Could you check a few things on this model? Use its own coordinates, in mm. A direction names the side the tool comes from. Round coordinates to 2 decimals unless told otherwise and drop trailing zeros. Loops run counter-clockwise (first coordinate to the right, second up) from the corner with the lowest first, then second, coordinate; pieces in that order, holes last.
from build123d import *

# Parameters (mm, degrees)
SKETCH_1_W                = 47
SKETCH_1_H                = 50
EXTRUDE_1_DEPTH           = 100
SKETCH_2_W                = 43
SKETCH_2_H                = 46
CUT_EXTRUDE_1_DEPTH       = 122.280666225
HOLE_WIZARD_1_D           = 2.4
HOLE_WIZARD_1_CSINK_D     = 4.5
HOLE_WIZARD_1_CSINK_ANGLE = 90
SKETCH_31_W               = 4
SKETCH_31_H               = 25
EXTRUDE_4_DEPTH           = 37
SKETCH_32_R               = 5
CUT_EXTRUDE_2_DEPTH       = 4
SKETCH_33_R               = 1.9
EXTRUDE_5_DEPTH           = 1.6
SKETCH_34_R               = 1.05
CUT_EXTRUDE_3_DEPTH       = 101.189819842
SKETCH_35_W               = 68
SKETCH_35_H               = 4
EXTRUDE_6_DEPTH           = 35
CUT_EXTRUDE_4_REACH       = 123.281
SKETCH_36_R               = 1.25
CUT_EXTRUDE_5_REACH       = 123.281
CUT_EXTRUDE_6_REACH       = 123.281
SKETCH_39_R               = 2.5
CUT_EXTRUDE_7_DEPTH       = 1.5
CUT_EXTRUDE_8_DEPTH       = 2
CUT_EXTRUDE_9_REACH       = 122.47
SKETCH_41_R               = 1.5
SKETCH_42_R               = 1.5
CUT_EXTRUDE_10_DEPTH      = 2
RIB_2_REACH               = 99.933
SKETCH_46_WALL_W          = 251.717080448
SKETCH_46_WALL_H          = 2
RIB_3_REACH               = 100.118
SKETCH_47_WALL_W          = 252.08841221
SKETCH_47_WALL_H          = 2
SKETCH_48_W               = 2
SKETCH_48_H               = 15
EXTRUDE_7_DEPTH           = 20
CUT_EXTRUDE_11_REACH      = 105.589


with BuildPart() as part:
    # 草图1 → 凸台-拉伸1 (new body)
    with BuildSketch(Plane(origin=(0, 0, 0), x_dir=(0, 0, -1), z_dir=(1, 0, 0))):
        with Locations((-23.5, 25)):
            Rectangle(SKETCH_1_W, SKETCH_1_H)
    extrude(amount=-EXTRUDE_1_DEPTH)

    # 草图2 → 切除-拉伸1 (cut, through all)
    with BuildSketch(Plane(origin=(0, 0, 0), x_dir=(0, 0, -1), z_dir=(1, 0, 0))):
        with Locations((-25.5, 23)):
            Rectangle(SKETCH_2_W, SKETCH_2_H)
    extrude(amount=-CUT_EXTRUDE_1_DEPTH, mode=Mode.SUBTRACT)

    # 打孔尺寸(%根据十字)槽沉头木螺钉的类型1 (through all)
    with Locations(Plane.XY.offset(4)):
        with Locations((-58, 26.5), (-50, 26.5), (-58, 18.5), (-50, 18.5), (-58, 10.5), (-50, 10.5), (-42, 10.5), (-42, 18.5), (-42, 26.5)):
            CounterSinkHole(HOLE_WIZARD_1_D / 2, HOLE_WIZARD_1_CSINK_D / 2, counter_sink_angle=HOLE_WIZARD_1_CSINK_ANGLE)

    # 草图31 → 凸台-拉伸4 (add)
    with BuildSketch(Plane(origin=(0, 0, 0), x_dir=(-1, 0, 0), z_dir=(0, 0, -1))):
        with Locations((23.4, 18.5)):
            Rectangle(SKETCH_31_W, SKETCH_31_H)
    extrude(amount=EXTRUDE_4_DEPTH)

    # 草图32 → 切除-拉伸2 (cut)
    with BuildSketch(Plane.ZY.offset(25.4)):
        with Locations((-26, 18.5)):
            Circle(SKETCH_32_R)
    extrude(amount=-CUT_EXTRUDE_2_DEPTH, mode=Mode.SUBTRACT)

    # 草图33 → 凸台-拉伸5 (add)
    with BuildSketch(Plane.ZY.offset(25.4)):
        with Locations(Location((-26, 26.5, 0), (0, 0, 180))):
            Circle(SKETCH_33_R)
        with Locations(Location((-18, 18.5, 0), (0, 0, 180))):
            Circle(SKETCH_33_R)
        with Locations(Location((-26, 10.5, 0), (0, 0, 180))):
            Circle(SKETCH_33_R)
        with Locations(Location((-34, 18.5, 0), (0, 0, 180))):
            Circle(SKETCH_33_R)
    extrude(amount=EXTRUDE_5_DEPTH)

    # 草图34 → 切除-拉伸3 (cut, through all)
    with BuildSketch(Plane.ZY.offset(27)):
        with Locations((-26, 26.5)):
            Circle(SKETCH_34_R)
        with Locations((-18, 18.5)):
            Circle(SKETCH_34_R)
        with Locations((-26, 10.5)):
            Circle(SKETCH_34_R)
        with Locations((-34, 18.5)):
            Circle(SKETCH_34_R)
    extrude(amount=-CUT_EXTRUDE_3_DEPTH, mode=Mode.SUBTRACT)

    # 草图35 → 凸台-拉伸6 (add)
    with BuildSketch(Plane(origin=(0, 0, 0), x_dir=(-1, 0, 0), z_dir=(0, 0, -1))):
        with Locations((50, 48)):
            Rectangle(SKETCH_35_W, SKETCH_35_H)
    extrude(amount=EXTRUDE_6_DEPTH)

    # 草图36 → 切除-拉伸4 (cut, up to next)
    with BuildSketch(Plane(origin=(0, 50, 0), x_dir=(1, 0, 0), z_dir=(0, 1, 0)), mode=Mode.PRIVATE) as cut_extrude_4_sk1:
        with Locations(Location((-78, 28, 0), (0, 0, 270))):
            Circle(SKETCH_36_R)
    cut_extrude_4_tool1 = extrude(cut_extrude_4_sk1.sketch, amount=-CUT_EXTRUDE_4_REACH, mode=Mode.PRIVATE) & part.part
    # 草图36 → 切除-拉伸4 (cut, up to next)
    with BuildSketch(Plane(origin=(0, 50, 0), x_dir=(1, 0, 0), z_dir=(0, 1, 0)), mode=Mode.PRIVATE) as cut_extrude_4_sk2:
        with Locations(Location((-22, 28, 0), (0, 0, 270))):
            Circle(SKETCH_36_R)
    cut_extrude_4_tool2 = extrude(cut_extrude_4_sk2.sketch, amount=-CUT_EXTRUDE_4_REACH, mode=Mode.PRIVATE) & part.part
    # 草图36 → 切除-拉伸4 (cut, up to next)
    with BuildSketch(Plane(origin=(0, 50, 0), x_dir=(1, 0, 0), z_dir=(0, 1, 0)), mode=Mode.PRIVATE) as cut_extrude_4_sk3:
        with Locations(Location((-70, -42, 0), (0, 0, 270))):
            Circle(SKETCH_36_R)
    cut_extrude_4_tool3 = extrude(cut_extrude_4_sk3.sketch, amount=-CUT_EXTRUDE_4_REACH, mode=Mode.PRIVATE) & part.part
    # 草图36 → 切除-拉伸4 (cut, up to next)
    with BuildSketch(Plane(origin=(0, 50, 0), x_dir=(1, 0, 0), z_dir=(0, 1, 0)), mode=Mode.PRIVATE) as cut_extrude_4_sk4:
        with Locations(Location((-30, -42, 0), (0, 0, 270))):
            Circle(SKETCH_36_R)
    cut_extrude_4_tool4 = extrude(cut_extrude_4_sk4.sketch, amount=-CUT_EXTRUDE_4_REACH, mode=Mode.PRIVATE) & part.part
    add(cut_extrude_4_tool1.solids().sort_by_distance((-78, 50, -28))[0], mode=Mode.SUBTRACT)
    add(cut_extrude_4_tool2.solids().sort_by_distance((-22, 50, -28))[0], mode=Mode.SUBTRACT)
    add(cut_extrude_4_tool3.solids().sort_by_distance((-70, 50, 42))[0], mode=Mode.SUBTRACT)
    add(cut_extrude_4_tool4.solids().sort_by_distance((-30, 50, 42))[0], mode=Mode.SUBTRACT)

    # 草图37 → 切除-拉伸5 (cut, up to next)
    with BuildSketch(Plane(origin=(0, 50, 0), x_dir=(1, 0, 0), z_dir=(0, 1, 0)), mode=Mode.PRIVATE) as cut_extrude_5_sk1:
        Polygon((-100, -47), (-80, -47), (-100, 0), align=None)
    cut_extrude_5_tool1 = extrude(cut_extrude_5_sk1.sketch, amount=-CUT_EXTRUDE_5_REACH, mode=Mode.PRIVATE) & part.part
    # 草图37 → 切除-拉伸5 (cut, up to next)
    with BuildSketch(Plane(origin=(0, 50, 0), x_dir=(1, 0, 0), z_dir=(0, 1, 0)), mode=Mode.PRIVATE) as cut_extrude_5_sk2:
        Polygon((0, -47), (-20, -47), (0, 0), align=None)
    cut_extrude_5_tool2 = extrude(cut_extrude_5_sk2.sketch, amount=-CUT_EXTRUDE_5_REACH, mode=Mode.PRIVATE) & part.part
    add(cut_extrude_5_tool1.solids().sort_by_distance((-93.333333, 50, 31.333333))[0], mode=Mode.SUBTRACT)
    add(cut_extrude_5_tool2.solids().sort_by_distance((-6.666667, 50, 31.333333))[0], mode=Mode.SUBTRACT)

    # 草图38 → 切除-拉伸6 (cut, up to next)
    with BuildSketch(Plane(origin=(0, 0, 0), x_dir=(-1, 0, 0), z_dir=(0, 0, -1)), mode=Mode.PRIVATE) as cut_extrude_6_sk1:
        Polygon((0, 0), (18, 0), (0, 50), align=None)
    cut_extrude_6_tool1 = extrude(cut_extrude_6_sk1.sketch, amount=-CUT_EXTRUDE_6_REACH, mode=Mode.PRIVATE) & part.part
    # 草图38 → 切除-拉伸6 (cut, up to next)
    with BuildSketch(Plane(origin=(0, 0, 0), x_dir=(-1, 0, 0), z_dir=(0, 0, -1)), mode=Mode.PRIVATE) as cut_extrude_6_sk2:
        Polygon((100, 0), (82, 0), (100, 50), align=None)
    cut_extrude_6_tool2 = extrude(cut_extrude_6_sk2.sketch, amount=-CUT_EXTRUDE_6_REACH, mode=Mode.PRIVATE) & part.part
    add(cut_extrude_6_tool1.solids().sort_by_distance((-6, 16.666667, 0))[0], mode=Mode.SUBTRACT)
    add(cut_extrude_6_tool2.solids().sort_by_distance((-94, 16.666667, 0))[0], mode=Mode.SUBTRACT)

    # 草图39 → 切除-拉伸7 (cut)
    with BuildSketch(Plane.XZ.offset(-46)):
        with Locations(Location((-70, 42, 0), (0, 0, 270))):
            Circle(SKETCH_39_R)
        with Locations(Location((-30, 42, 0), (0, 0, 270))):
            Circle(SKETCH_39_R)
        with Locations(Location((-78, -28, 0), (0, 0, 270))):
            Circle(SKETCH_39_R)
        with Locations(Location((-22, -28, 0), (0, 0, 270))):
            Circle(SKETCH_39_R)
    extrude(amount=-CUT_EXTRUDE_7_DEPTH, mode=Mode.SUBTRACT)

    # 草图40 → 切除-拉伸8 (cut)
    with BuildSketch(Plane(origin=(0, 50, 0), x_dir=(1, 0, 0), z_dir=(0, 1, 0))):
        Polygon((-79.75, 24.5), (-60, 24.5), (-60, 35), (-40, 35), (-40, 24.5), (-20.25, 24.5), (-20.25, -21.6), (-79.75, -21.6), align=None)
    extrude(amount=-CUT_EXTRUDE_8_DEPTH, mode=Mode.SUBTRACT)

    # 草图41 → 切除-拉伸9 (cut, up to next)
    with BuildSketch(Plane(origin=(0, 48, 0), x_dir=(1, 0, 0), z_dir=(0, 1, 0)), mode=Mode.PRIVATE) as cut_extrude_9_sk1:
        with Locations(Location((-74.75, 14.5, 0), (0, 0, 270))):
            Circle(SKETCH_41_R)
    cut_extrude_9_tool1 = extrude(cut_extrude_9_sk1.sketch, amount=-CUT_EXTRUDE_9_REACH, mode=Mode.PRIVATE) & part.part
    # 草图41 → 切除-拉伸9 (cut, up to next)
    with BuildSketch(Plane(origin=(0, 48, 0), x_dir=(1, 0, 0), z_dir=(0, 1, 0)), mode=Mode.PRIVATE) as cut_extrude_9_sk2:
        with Locations(Location((-74.75, -11.6, 0), (0, 0, 270))):
            Circle(SKETCH_41_R)
    cut_extrude_9_tool2 = extrude(cut_extrude_9_sk2.sketch, amount=-CUT_EXTRUDE_9_REACH, mode=Mode.PRIVATE) & part.part
    # 草图41 → 切除-拉伸9 (cut, up to next)
    with BuildSketch(Plane(origin=(0, 48, 0), x_dir=(1, 0, 0), z_dir=(0, 1, 0)), mode=Mode.PRIVATE) as cut_extrude_9_sk3:
        with Locations(Location((-25.25, 14.5, 0), (0, 0, 270))):
            Circle(SKETCH_41_R)
    cut_extrude_9_tool3 = extrude(cut_extrude_9_sk3.sketch, amount=-CUT_EXTRUDE_9_REACH, mode=Mode.PRIVATE) & part.part
    # 草图41 → 切除-拉伸9 (cut, up to next)
    with BuildSketch(Plane(origin=(0, 48, 0), x_dir=(1, 0, 0), z_dir=(0, 1, 0)), mode=Mode.PRIVATE) as cut_extrude_9_sk4:
        with Locations(Location((-25.25, -11.6, 0), (0, 0, 270))):
            Circle(SKETCH_41_R)
    cut_extrude_9_tool4 = extrude(cut_extrude_9_sk4.sketch, amount=-CUT_EXTRUDE_9_REACH, mode=Mode.PRIVATE) & part.part
    add(cut_extrude_9_tool1.solids().sort_by_distance((-74.75, 48, -14.5))[0], mode=Mode.SUBTRACT)
    add(cut_extrude_9_tool2.solids().sort_by_distance((-74.75, 48, 11.6))[0], mode=Mode.SUBTRACT)
    add(cut_extrude_9_tool3.solids().sort_by_distance((-25.25, 48, -14.5))[0], mode=Mode.SUBTRACT)
    add(cut_extrude_9_tool4.solids().sort_by_distance((-25.25, 48, 11.6))[0], mode=Mode.SUBTRACT)

    # 草图42 → 切除-拉伸10 (cut)
    with BuildSketch(Plane(origin=(0, 48, 0), x_dir=(1, 0, 0), z_dir=(0, 1, 0))):
        with Locations(Location((-62.07, 16.5, 0), (0, 0, 270))):
            Circle(SKETCH_42_R)
        with Locations(Location((-37.93, 16.5, 0), (0, 0, 270))):
            Circle(SKETCH_42_R)
        with Locations(Location((-37.93, -9.5, 0), (0, 0, 270))):
            Circle(SKETCH_42_R)
        with Locations(Location((-62.07, -9.5, 0), (0, 0, 270))):
            Circle(SKETCH_42_R)
    extrude(amount=-CUT_EXTRUDE_10_DEPTH, mode=Mode.SUBTRACT)

    # 草图46 wall → 筋2 (add, up to next)
    with BuildSketch(Plane(origin=(-30.13, 23, 18), x_dir=(0, -0.854198555614, -0.519946946896), z_dir=(0, 0.519946946896, -0.854198555614)), mode=Mode.PRIVATE) as rib_2_sk1:
        with Locations((0, 1)):
            Rectangle(SKETCH_46_WALL_W, SKETCH_46_WALL_H)
    rib_2_tool1 = extrude(rib_2_sk1.sketch, amount=RIB_2_REACH, mode=Mode.PRIVATE) - part.part
    add(rib_2_tool1.solids().sort_by_distance((-30.13, 23, 18))[0])

    # 草图47 wall → 筋3 (add, up to next)
    with BuildSketch(Plane(origin=(-70.13, 23, 18), x_dir=(0, -0.854198555614, -0.519946946896), z_dir=(0, 0.519946946896, -0.854198555614)), mode=Mode.PRIVATE) as rib_3_sk1:
        with Locations((0, -1)):
            Rectangle(SKETCH_47_WALL_W, SKETCH_47_WALL_H)
    rib_3_tool1 = extrude(rib_3_sk1.sketch, amount=RIB_3_REACH, mode=Mode.PRIVATE) - part.part
    add(rib_3_tool1.solids().sort_by_distance((-70.13, 23, 18))[0])

    # 草图48 → 凸台-拉伸7 (add)
    with BuildSketch(Plane(origin=(0, 0, 0), x_dir=(-1, 0, 0), z_dir=(0, 0, -1))):
        with Locations((23.4, 38.5)):
            Rectangle(SKETCH_48_W, SKETCH_48_H)
    extrude(amount=EXTRUDE_7_DEPTH)

    # 草图49 → 切除-拉伸11 (cut, up to next)
    with BuildSketch(Plane(origin=(-22.4, 0, 0), x_dir=(0, 0, -1), z_dir=(1, 0, 0)), mode=Mode.PRIVATE) as cut_extrude_11_sk1:
        Polygon((5, 46), (20, 46), (20, 31), align=None)
    cut_extrude_11_tool1 = extrude(cut_extrude_11_sk1.sketch, amount=-CUT_EXTRUDE_11_REACH, mode=Mode.PRIVATE) & part.part
    add(cut_extrude_11_tool1.solids().sort_by_distance((-22.4, 41, -15))[0], mode=Mode.SUBTRACT)


solid = part.part
Item 1: If we section it at B-B, the plane z = 42: Please give me the cut outline in (x, y), then the cut area to 3 significant figures.
Results list:
outline: (-82.13, 46) - (-72.5, 46) - (-72.5, 47.5) - (-71.25, 47.5) - (-71.25, 50) - (-82.13, 50) - close; (-68.75, 47.5) - (-67.5, 47.5) - (-67.5, 46) - (-32.5, 46) - (-32.5, 47.5) - (-31.25, 47.5) - (-31.25, 50) - (-68.75, 50) - close; (-28.75, 47.5) - (-27.5, 47.5) - (-27.5, 46) - (-17.87, 46) - (-17.87, 50) - (-28.75, 50) - close
area: 230 mm2
Item 2: If we section it at A-A, the plane x = -42: Please give me the cut outline in (y, z), then the cut area to 3 significant figures.
Results list:
outline: (0, 0) - (9.3, 0) - (9.3, 2.95) - (8.25, 4) - (0, 4) - close; (11.7, 0) - (17.3, 0) - (17.3, 2.95) - (16.25, 4) - (12.75, 4) - (11.7, 2.95) - close; (19.7, 0) - (25.3, 0) - (25.3, 2.95) - (24.25, 4) - (20.75, 4) - (19.7, 2.95) - close; (27.7, 0) - (46, 0) - (46, -35) - (48, -35) - (48, 21.6) - (50, 21.6) - (50, 47) - (46, 47) - (46, 4) - (28.75, 4) - (27.7, 2.95) - close
area: 367 mm2
Item 3: If I drill on line 1 along Y through (x, z) = (-25.15, -26); line 2 along X through (y, z) = (45.5, 7); line 3 along X through (y, z) = (26.5, 2.3), over which ranges is the centre line in solid material (lowest first)?
Results list:
line 1: y = 6 to 9.45, 11.55 to 13.5, 23.5 to 25.45, 27.55 to 31, 46 to 50
line 2: x = -70.13 to -68.13, -32.13 to -30.13
line 3: x = -91.54 to -59.2, -56.8 to -51.2, -48.8 to -43.2, -40.8 to -8.46
Item 4: We'd pull the mould along X, two halves only. Please class faces 1 (the flat face through (-25.4, 18, -14)), 2 (the flat face through (-68.13, 33, 14)), 3 (the cylindrical face through (-23.4, 15.5, -30)): released by +X, released by -X, zero draft, split by the parting line, or undercut.
Results list:
face 1: released by -X
face 2: undercut
face 3: zero draft
Item 5: Will these pins go through, and if not, where does the flat tip stop? pin 1 (2.5 mm diameter, centred on x = -25.25, z = -14.5, fed in from -Y); pin 2 (6 mm diameter, centred on x = -84.5, y = 28, fed in from +Z); pin 3 (5 mm diameter, centred on x = -11.5, z = 19, fed in from -Y); pin 4 (2 mm diameter, centred on x = -42, y = 26.5, fed in from +Z).
Results list:
pin 1: stops at y = 6
pin 2: stops at z = 4
pin 3: stops at y = 46
pin 4: passes through
Item 6: If we section it at D-D, the plane z = 19: Please give me the cut outline in (x, y).
Results list:
outline: (-91.91, 46) - (-70.13, 46) - (-70.13, 24.64) - (-68.13, 24.64) - (-68.13, 46) - (-32.13, 46) - (-32.13, 24.64) - (-30.13, 24.64) - (-30.13, 46) - (-8.09, 46) - (-8.09, 50) - (-20.25, 50) - (-20.25, 48) - (-79.75, 48) - (-79.75, 50) - (-91.91, 50) - close
Item 7: For faces 4 (the flat face through (-50, 23, 4)), 5 (the cylindrical face through (-24.239, 25.568, -25.515)), 6 (the flat face through (-27, 28, -26)), 7 (the cylindrical face through (-80.44, 46.74, -27.46)), 8 (the flat face through (-23, 6, -18)), which set-ups out of +Z, -Z, +X, -X, +Y, -Y let a thin tool reach every point of the face, with its end or its side?
Results list:
face 4: +Z, -Y
face 5: +X, -X
face 6: -Z, -X, -Y
face 7: -Y
face 8: -Z, +X, -X, -Y
Item 8: If we section it at C-C, the plane z = 30.5: Please give me the cut outline in (x, y), then the cut area to 3 significant figures.
Results list:
outline: (-87.02, 46) - (-70.13, 46) - (-70.13, 43.54) - (-68.13, 43.54) - (-68.13, 46) - (-32.13, 46) - (-32.13, 43.54) - (-30.13, 43.54) - (-30.13, 46) - (-12.98, 46) - (-12.98, 50) - (-87.02, 50) - close
area: 306 mm2
